Verification items for the finished model (mm, model axes). A direction names the side the tool comes from. Give positions to 0.01 mm unless a question says otherwise; leave off trailing zeros. Loops run counter-clockwise (first coordinate to the right, second up) from the corner with the lowest first, then second, coordinate; pieces in that order, holes last. Notation, with made-up numbers: (37, -34) - (42, -34) arc R6 cw to (42, -27) - close; hole circle Ø5 at (49.5, 17.25). An arc over 180 degrees is marked (long way). One line per item, written item: value. Start each with the question number.
1. Sectioned sample at B-B (x = -8). Record the cut outline in (y, z).
2. Sectioned sample at C-C (y = 8.25). Record the cut outline in (x, z), plus the area to 3 significant figures.
3. Sectioned sample at D-D (z = 4.75). Record the cut outline in (x, y), plus the area to 3 significant figures.
4. Gauge pin test, flat ends, axial feed: pin 1 (1.6 mm diameter, centred on y = -0.5, z = 3, fed in from +X); pin 2 (8 mm diameter, centred on x = -4, y = 5.5, fed in from -Z); pin 3 (1.5 mm diameter, centred on x = -8, z = 11, fed in from -Y); pin 4 (3 mm diameter, centred on x = -12, y = -1, fed in from +Z). Record the tip position at first contact, or that the pin passes through.
5. Mould release check, pull along X, two halves, no side actions. Record for faces 1 (the flat face through (-9.4, 14.8, 12)), 2 (the flat face through (3, -1.8, 2)), 3 (the flat face through (-4, 7.35, 6)): pulls with the +X half, pulls with the -X half, needs draft (parallel to the pull), parting line crosses it, or undercut.
6. Scan lines: L1, parallel to X at y = -1.75, z = 4.25; L2, parallel to Y at x = 2.5, z = 9.5; L3, parallel to Z at x = -11.5, y = 4. Record each from-to range of solid material in increasing order. Write a range as [from, to].
7. Sectioned sample at A-A (y = -0.25). Record the cut outline in (x, z).
8. Access from +Z, -Z, +X, -X, +Y, -Y to the whole of each face (thin tool, end or side, straight path). Record for faces 4 (the flat face through (2, -2, 5)), 5 (the flat face through (-11, 9, 2)), 6 (the cylindrical face through (-10.94, 6.97, 2.46)).
from build123d import *

# Parameters (mm, degrees)
PAD017_DEPTH           = 5
PAD020_DEPTH           = 6.25
SKETCH038_W            = 10
SKETCH038_H            = 1.65
PAD021_DEPTH           = 5
SKETCH097_W            = 12.5
SKETCH097_H            = 1.65
PAD066_DEPTH           = 12.5
SKETCH094_W            = 12.5
SKETCH094_H            = 1.65
PAD067_DEPTH           = 9.6
SKETCH095_W            = 9.6
SKETCH095_H            = 1.65
PAD068_DEPTH           = 12.5
SKETCH096_W            = 12.5
SKETCH096_H            = 1.65
PAD069_DEPTH           = 12.5
LINEARPATTERN022_COUNT = 2
LINEARPATTERN022_PITCH = 3.3
CHAMFER012_SIZE        = 1


with BuildPart() as obj1:
    # Sketch034 → Pad017 (new body)
    with BuildSketch(Plane.XY):
        with BuildLine():
            Line((-1.35, -1.8), (-1.35, 6))
            ThreePointArc((0, 7.35), (-0.954594, 6.954594), (-1.35, 6))
            Line((0, 9), (0, 7.35))
            Line((-2.6, 9), (0, 9))
            Line((-2.6, -1.8), (-2.6, 9))
            Line((-3.85, -1.8), (-2.6, -1.8))
            ThreePointArc((-3.85, -1.8), (-3.439949, -2.789949), (-2.45, -3.2))
            Line((-1.35, -3.2), (-2.45, -3.2))
            Line((-1.35, -1.8), (-1.35, -3.2))
        make_face()
    extrude(amount=PAD017_DEPTH)

    # Sketch037 → Pad020 (join)
    with BuildSketch(Plane.XY):
        Polygon((-1.35, 0.2), (-1.35, 1.6), (-2.6, 1.6), (-3.85, 1.6), (-3, 0.2), (-2.6, 0.2), align=None)
    extrude(amount=PAD020_DEPTH)


with BuildPart() as body035:
    # Mirror002: instance of _obj1
    add(obj1.part.mirror(Plane(origin=(5, 0, 0), x_dir=(0, 1, 0), z_dir=(-1, 0, 0))))

    # Fusion002: union _obj1
    add(obj1.part)


with BuildPart() as body035_1:
    # Clone003 placement: moved
    add(body035.part.moved(Location((-5, 0, 0))))

    # Sketch038 → Pad021 (new body)
    with BuildSketch(Plane.XY):
        with Locations((0, 8.175)):
            Rectangle(SKETCH038_W, SKETCH038_H)
    extrude(amount=PAD021_DEPTH)

    # Sketch097 → Pad066 (new body)
    with BuildSketch(Plane.XY):
        with Locations((1.35, 8.175)):
            Rectangle(SKETCH097_W, SKETCH097_H)
    extrude(amount=PAD066_DEPTH)

    # Sketch094 → Pad067 (join)
    with BuildSketch(Plane.XY):
        with Locations((1.35, 9.825)):
            Rectangle(SKETCH094_W, SKETCH094_H)
    pad067 = extrude(amount=PAD067_DEPTH)

    # Sketch095 → Pad068 (join)
    with BuildSketch(Plane.XY):
        with Locations((2.8, 9.825)):
            Rectangle(SKETCH095_W, SKETCH095_H)
    pad068 = extrude(amount=PAD068_DEPTH)

    # Sketch096 → Pad069 (join)
    with BuildSketch(Plane.XY):
        with Locations((1.35, 11.475)):
            Rectangle(SKETCH096_W, SKETCH096_H)
    pad069 = extrude(amount=PAD069_DEPTH)

    # LinearPattern022: Pad069, Pad068, Pad067 ×2
    with Locations(*[(0, i * LINEARPATTERN022_PITCH, 0) for i in range(1, LINEARPATTERN022_COUNT)]):
        add(pad069)
        add(pad068)
        add(pad067)

    # Chamfer012
    chamfer012_edges = [body035_1.edges().sort_by_distance(p)[0] for p in [
        (-4.9, 8.175, 12.5),
        (-4.9, 11.475, 12.5),
        (-4.9, 14.775, 12.5),
    ]]
    chamfer(chamfer012_edges, length=CHAMFER012_SIZE)


with BuildPart() as body035_2:
    # Body035 placement: moved
    add(body035_1.part.moved(Location((-5, 0, 0))))


solid = body035_2.part
Results are:
1. outline: (7.35, 0) - (15.6, 0) - (15.6, 12.5) - (13.95, 12.5) - (13.95, 9.6) - (12.3, 9.6) - (12.3, 12.5) - (10.65, 12.5) - (10.65, 9.6) - (9, 9.6) - (9, 12.5) - (7.35, 12.5) - close
2. outline: (-12.6, 0) - (2.6, 0) - (2.6, 12.5) - (-8.9, 12.5) - (-9.9, 11.5) - (-9.9, 5) - (-12.6, 5) - close
2. area: 169 mm^2
3. outline: (-13.85, -1.8) arc R1.4 ccw to (-12.45, -3.2) - (-11.35, -3.2) - (-11.35, 6) arc R1.35 cw to (-10, 7.35) - (0, 7.35) arc R1.35 cw to (1.35, 6) - (1.35, -3.2) - (2.45, -3.2) arc R1.4 ccw to (3.85, -1.8) - (2.6, -1.8) - (2.6, 0.2) - (3, 0.2) - (3.85, 1.6) - (2.6, 1.6) - (2.6, 15.6) - (-9.9, 15.6) - (-9.9, 9) - (-12.6, 9) - (-12.6, 1.6) - (-13.85, 1.6) - (-13, 0.2) - (-12.6, 0.2) - (-12.6, -1.8) - close
3. area: 140 mm^2
4. pin 1: stops at x = 3.06
4. pin 2: stops at z = 0
4. pin 3: stops at y = 7.35
4. pin 4: stops at z = 6.25
5. face 1: pulls with the -X half
5. face 2: needs draft
5. face 3: undercut
6. L1: x = [-12.6, -11.35], [1.35, 2.6]
6. L2: y = [7.35, 15.6]
6. L3: z = [0, 5]
7. outline: (-12.6, 0) - (-11.35, 0) - (-11.35, 5) - (-12.6, 5) - close; (1.35, 0) - (2.6, 0) - (2.6, 5) - (1.35, 5) - close
8. face 4: +Z, +X, -X, -Y
8. face 5: +Z, -Z, -X, +Y
8. face 6: +Z, -Z, -Y
